Can you work these out from the model? Positions are in its coordinate system, mm. Face numbers are marked on the shaded views. A direction names the side the tool comes from. Coordinates: 2 decimals unless noted, no trailing zeros. Write each loop counter-clockwise with the first axis right and the second up, starting at its lowest first coordinate (ties: lowest second). Pieces come first, ordered by that corner, then holes. Notation, with made-up numbers: (89.5, 23.25) - (113.5, 23.25) arc R25 ccw to (113.5, 42.25) - close; hole circle Ø3 at (76, 59.5). An arc over 180 degrees is marked (long way). One line per question, with ' | ' between items. Start each with the question number.
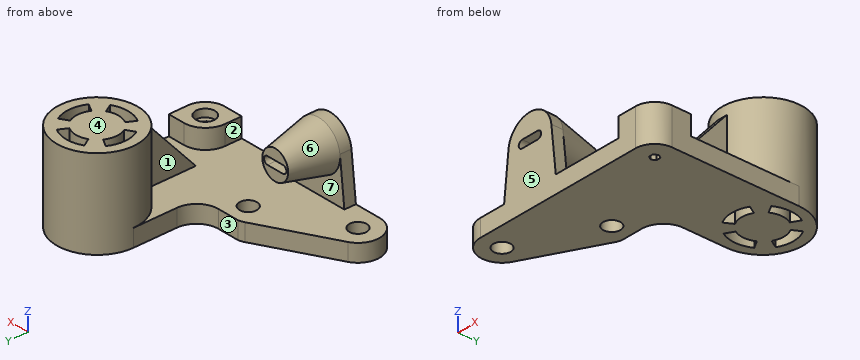
from build123d import *

# Parameters (mm, degrees)
IZIM1_R                     = 9
Y_KSEKLIK_EKSTR_ZYON1_DEPTH = 18
IZIM2_R                     = 42
Y_KSEKLIK_EKSTR_ZYON2_DEPTH = 92
Y_KSEKLIK_EKSTR_ZYON3_DEPTH = 20
KES_EKSTR_ZYON1_DEPTH       = 60
KES_EKSTR_ZYON2_DEPTH       = 108
FEDER1_REACH                = 282.501
IZIM6_WALL_W                = 648.043161204
IZIM6_WALL_H                = 10
Y_KSEKLIK_EKSTR_ZYON4_DEPTH = 12
IZIM9_R                     = 25
IZIM8_R                     = 15
KES_EKSTR_ZYON3_DEPTH       = 65
IZIM11_R                    = 10
KES_EKSTR_ZYON4_DEPTH       = 8


with BuildPart() as part:
    # Çizim1 → Yükseklik-Ekstrüzyon1 (new body)
    with BuildSketch(Plane.XY):
        with BuildLine():
            Line((-32.411549897, 0), (147.588450103, 0))
            ThreePointArc((147.588450103, 0), (161.730585727, 5.857864376), (167.588450103, 20))
            Line((167.588450103, 20), (167.588450103, 152))
            ThreePointArc((167.588450103, 152), (125.588450103, 110), (83.588450103, 152))
            Line((83.588450103, 152), (83.588450103, 106.718465751))
            ThreePointArc((83.588450103, 106.718465751), (76.934365543, 90.65408456), (60.869984352, 84))
            Line((60.869984352, 84), (38.285308022, 84))
            ThreePointArc((38.285308022, 84), (35.198315251, 83.226334615), (32.273122012, 81.972808782))
            Line((32.273122012, 81.972808782), (-42.891293999, 42.41042349))
            ThreePointArc((-42.891293999, 42.41042349), (-54.25456398, 17.102525059), (-32.411549897, 0))
        make_face()
        with Locations((48.588450103, 64)):
            Circle(IZIM1_R, mode=Mode.SUBTRACT)
        with Locations((-32.411549897, 22.5)):
            Circle(IZIM1_R, mode=Mode.SUBTRACT)
    extrude(amount=Y_KSEKLIK_EKSTR_ZYON1_DEPTH)

    # Çizim2 → Yükseklik-Ekstrüzyon2 (add)
    with BuildSketch(Plane.XY):
        with Locations((125.588450103, 152)):
            Circle(IZIM2_R)
    extrude(amount=Y_KSEKLIK_EKSTR_ZYON2_DEPTH)

    # Çizim3 → Yükseklik-Ekstrüzyon3 (add)
    with BuildSketch(Plane.XY.offset(18)):
        with BuildLine():
            Line((127.588450103, 0), (127.588450103, 17.51012232))
            ThreePointArc((127.588450103, 17.51012232), (134.175582768, 33.412867336), (150.078327783, 40))
            Line((150.078327783, 40), (167.588450103, 40))
            Line((167.588450103, 40), (167.588450103, 20))
            ThreePointArc((167.588450103, 20), (161.730585727, 5.857864376), (147.588450103, 0))
            Line((147.588450103, 0), (127.588450103, 0))
        make_face()
    extrude(amount=Y_KSEKLIK_EKSTR_ZYON3_DEPTH)

    # Çizim4 → Kes-Ekstrüzyon1 (cut)
    with BuildSketch(Plane.XY.offset(38)):
        Polygon((145.407352826, 15.928618416), (150.023821345, 16.075423558), (152.204918622, 20.146805142), (149.76954738, 24.071381584), (145.153078862, 23.924576442), (142.971981585, 19.853194858), align=None)
    extrude(amount=-KES_EKSTR_ZYON1_DEPTH, mode=Mode.SUBTRACT)

    # Çizim5 → Kes-Ekstrüzyon2 (cut)
    with BuildSketch(Plane.XY.offset(92)):
        with BuildLine():
            Line((136.588450103, 171.052558883), (141.588450103, 179.712812921))
            ThreePointArc((141.588450103, 179.712812921), (125.588450103, 184), (109.588450103, 179.712812921))
            Line((109.588450103, 179.712812921), (114.588450103, 171.052558883))
            ThreePointArc((114.588450103, 171.052558883), (125.588450103, 174), (136.588450103, 171.052558883))
        make_face()
        with BuildLine():
            Line((144.641008987, 141), (153.301263025, 136))
            ThreePointArc((153.301263025, 136), (157.588450103, 152), (153.301263025, 168))
            Line((153.301263025, 168), (144.641008987, 163))
            ThreePointArc((144.641008987, 163), (147.588450103, 152), (144.641008987, 141))
        make_face()
        with BuildLine():
            Line((114.588450103, 132.947441117), (109.588450103, 124.287187079))
            ThreePointArc((109.588450103, 124.287187079), (125.588450103, 120), (141.588450103, 124.287187079))
            Line((141.588450103, 124.287187079), (136.588450103, 132.947441117))
            ThreePointArc((136.588450103, 132.947441117), (125.588450103, 130), (114.588450103, 132.947441117))
        make_face()
        with BuildLine():
            Line((106.53589122, 163), (97.875637182, 168))
            ThreePointArc((97.875637182, 168), (93.588450103, 152), (97.875637182, 136))
            Line((97.875637182, 136), (106.53589122, 141))
            ThreePointArc((106.53589122, 141), (103.588450103, 152), (106.53589122, 163))
        make_face()
    extrude(amount=-KES_EKSTR_ZYON2_DEPTH, mode=Mode.SUBTRACT)

    # Çizim6 wall → Feder1 (add, up to next)
    with BuildSketch(Plane(origin=(125.59, 82, 50), x_dir=(0, -0.658504607869, -0.752576694707), z_dir=(0, 0.752576694707, -0.658504607869)), mode=Mode.PRIVATE) as feder1_sk1:
        Rectangle(IZIM6_WALL_W, IZIM6_WALL_H)
    feder1_tool1 = extrude(feder1_sk1.sketch, amount=FEDER1_REACH, mode=Mode.PRIVATE) - part.part
    add(feder1_tool1.solids().sort_by_distance((125.59, 82, 50))[0])

    # Çizim7 → Yükseklik-Ekstrüzyon4 (add)
    with BuildSketch(Plane(origin=(0, 0, 0), x_dir=(1, 0, 0), z_dir=(0, 1, 0))):
        with BuildLine():
            Line((-4.911549897, -18), (0.232687834, -65.681619291))
            ThreePointArc((0.232687834, -65.681619291), (25.088450103, -88), (49.944212373, -65.681619291))
            Line((49.944212373, -65.681619291), (55.088450103, -18))
            Line((55.088450103, -18), (-4.911549897, -18))
        make_face()
    extrude(amount=Y_KSEKLIK_EKSTR_ZYON4_DEPTH)

    # Çizim9 → Loft1 section 0
    with BuildSketch(Plane(origin=(0, 12, 0), x_dir=(1, 0, 0), z_dir=(0, 1, 0))):
        with Locations((25.088450103, -63)):
            Circle(IZIM9_R)
    # Çizim8 → Loft1 section 1
    with BuildSketch(Plane(origin=(0, 57, 0), x_dir=(1, 0, 0), z_dir=(0, 1, 0))):
        with Locations((25.088450103, -63)):
            Circle(IZIM8_R)
    loft()

    # Çizim10 → Kes-Ekstrüzyon3 (cut)
    with BuildSketch(Plane(origin=(0, 57, 0), x_dir=(1, 0, 0), z_dir=(0, 1, 0))):
        with BuildLine():
            Line((16.088450103, -59), (34.088450103, -59))
            ThreePointArc((34.088450103, -59), (38.088450103, -63), (34.088450103, -67))
            Line((34.088450103, -67), (16.088450103, -67))
            ThreePointArc((16.088450103, -67), (12.088450103, -63), (16.088450103, -59))
        make_face()
    extrude(amount=-KES_EKSTR_ZYON3_DEPTH, mode=Mode.SUBTRACT)

    # Çizim11 → Kes-Ekstrüzyon4 (cut)
    with BuildSketch(Plane.XY.offset(38)):
        with Locations((147.588450103, 20)):
            Circle(IZIM11_R)
    extrude(amount=-KES_EKSTR_ZYON4_DEPTH, mode=Mode.SUBTRACT)


solid = part.part
(1) If I drill on probe 1 along Y at (x, z) = (125, 51) (3 decimals); probe 2 along Y at (x, z) = (124.5, 36); probe 3 along Z at (x, y) = (26, 49.5), over which ranges is the centre line in solid material (lowest first)?
(2) If we mould it in two halves opening along Z, with no side actions, what happens to the marked faces 4, 5, 6 and 7? For each: +Z half, -Z half, draft (parallel to the pull), parting line (faces both ways), or undercut.
(3) If we section it at A-A on z = 35.5: Give the number of separate pieces and of enclosed holes in the cut face, plus the area to 3 significant figures.
(4) If we section it at B-B on y = 64: List the corners of the cut face in (x, z) for me.
(5) Which directions (+Z, -Z, +X, -X, +Y, -Y) give clear straight access to the entire face, cutting with the end or side of a thin tool? Please do the marked faces 1, 2 and 3.
(6) I'm going to push flat-ended pins straight in: pin 1 (24 mm diameter, centred on x = 27, z = 59.5, fed in from +Y); pin 2 (17 mm diameter, centred on y = 87.5, z = 57.5, fed in from +X); pin 3 (16 mm diameter, centred on x = -32.41, y = 22.5, fed in from +Z); pin 4 (1 mm diameter, centred on x = 94, z = 43, fed in from -Y). Where does each tip first touch, or does it pass through?
(7) If we section it at C-C on x = -35: List the corners of the cut face in (y, z) for me.
Values:
1) probe 1: 82.875 to 120.005, 130.008 to 173.992, 183.995 to 193.996 | probe 2: 69.75 to 120.02, 130.03 to 173.97, 183.98 to 193.99 | probe 3: 0 to 18, 46.36 to 59, 67 to 79.64
2) face 4: +Z half | face 5: draft | face 6: undercut | face 7: undercut
3) separate pieces: 3 | enclosed holes: 5 | area: 6,580 mm2
4) outline: (-1.87, 0) - (39.59, 0) - (39.59, 18) - (-1.87, 18) - close; (57.59, 0) - (167.59, 0) - (167.59, 18) - (130.59, 18) - (130.59, 29.43) - (120.59, 29.43) - (120.59, 18) - (57.59, 18) - close
5) face 1: +Z, -X, -Y | face 2: +Z, -Y | face 3: +Z, -Z, -X, +Y
6) pin 1: y = 57 | pin 2: x = 130.59 | pin 3: through | pin 4: y = 123.76
7) outline: (0.15, 0) - (13.88, 0) - (13.88, 18) - (0.15, 18) - close; (31.12, 0) - (46.56, 0) - (46.56, 18) - (31.12, 18) - close
